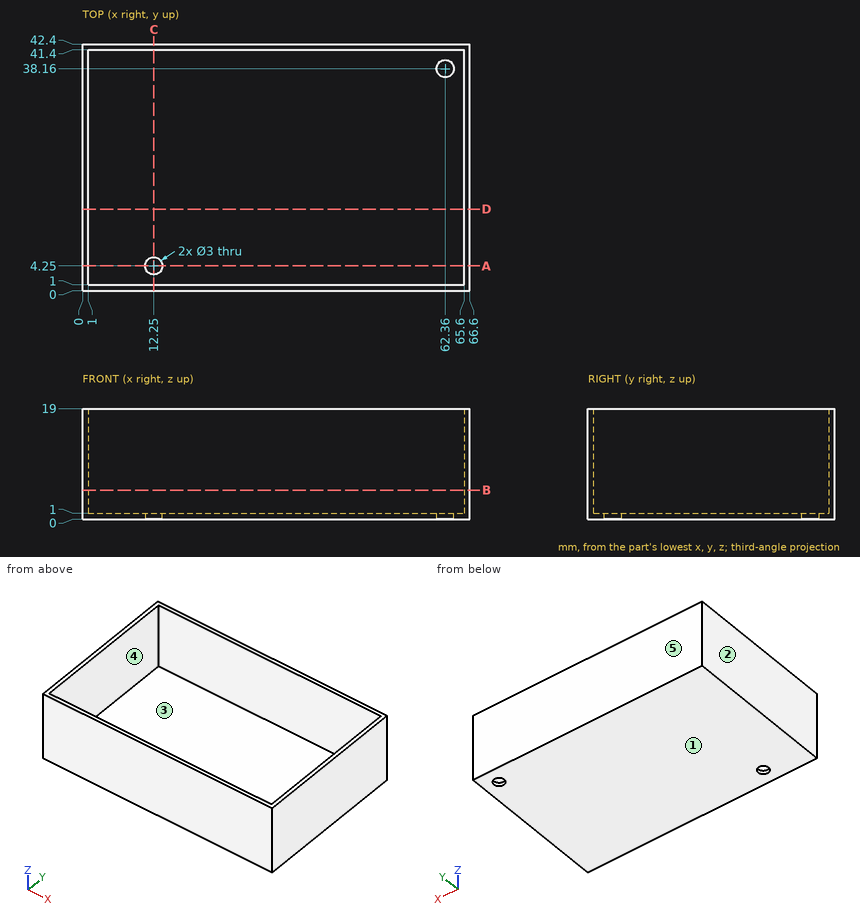
Could you check a few things on this drawing? It's one solid part, dimensions in mm from its lowest x, y, z. A direction names the side the tool comes from. Give positions to 0.01 mm unless a question says otherwise; leave off trailing zeros. Order: outer loops, then holes, each group sorted by start corner. A loop starts at its lowest first (then second) coordinate and runs counter-clockwise, first axis right, second up. Notation, with made-up numbers: M -16,85.5 L 17,85.5 A24 cw 17,123.5 Z; hole C 78.25,65 d2. An arc over 180 degrees is marked long. Use one line per item in the form item = value. Start each with the question number.
Item 1: If we section it at A-A (y = 4.25): Write out the boundary of the cut face in (x, z).
Item 2: We'd pull the mould along X, two halves only. Please class the marked faces 1, 2 and 3: +X half, -X half, draft (parallel to the pull), parting line (faces both ways), or undercut.
Item 3: If we section it at C-C (x = 12.25): Write out the boundary of the cut face in (y, z), then the cut area to 3 significant figures.
Item 4: Will this pin go through, and if not, where does the flat tip stop? pin 1 Ø5 at (x, y) = (62.36, 38.16) entering from +Z.
Item 5: If we section it at B-B (z = 5): Write out the boundary of the cut face in (x, y).
Item 6: If we section it at D-D (y = 14): Write out the boundary of the cut face in (x, z), then the cut area to 3 significant figures.
Item 7: For the marked faces 4 and 5, which set-ups out of +Z, -Z, +X, -X, +Y, -Y let a thin tool reach every point of the face, with its end or its side?
Item 8: If I drill on line 1 along Y through (x, z) = (12.25, 0.5); line 2 along X through (y, z) = (35.5, 17); line 3 along Y through (x, z) = (16.5, 14), over which ranges is the centre line in solid material (lowest first)?
Outcome:
q1.outline = M 0,0 L 10.75,0 L 10.75,1 L 1,1 L 1,19 L 0,19 Z; M 13.75,0 L 66.6,0 L 66.6,19 L 65.6,19 L 65.6,1 L 13.75,1 Z
q2.face_1 = draft
q2.face_2 = -X half
q2.face_3 = undercut
q3.outline = M 0,0 L 2.75,0 L 2.75,1 L 1,1 L 1,19 L 0,19 Z; M 5.75,0 L 42.4,0 L 42.4,19 L 41.4,19 L 41.4,1 L 5.75,1 Z
q3.area = 75.4 mm2
q4.pin_1 = 1
q5.outline = M 0,0 L 66.6,0 L 66.6,42.4 L 0,42.4 Z; hole M 1,1 L 65.6,1 L 65.6,41.4 L 1,41.4 Z
q6.outline = M 0,0 L 66.6,0 L 66.6,19 L 65.6,19 L 65.6,1 L 1,1 L 1,19 L 0,19 Z
q6.area = 103 mm2
q7.face_4 = +Z
q7.face_5 = +Z, -Z, +X, -X, +Y
q8.line_1 = 0 to 2.75, 5.75 to 42.4
q8.line_2 = 0 to 1, 65.6 to 66.6
q8.line_3 = 0 to 1, 41.4 to 42.4
